Verification items for the finished model (mm, model axes). A direction names the side the tool comes from. Give positions to 0.01 mm unless a question says otherwise; leave off trailing zeros. Order: outer loops, then holes, each group sorted by start corner. A loop starts at its lowest first (then second) coordinate and runs counter-clockwise, first axis right, second up. Notation, with made-up numbers: M 83,-7 L 123,-7 A21 cw 123,-2 Z; hole C 36.25,11 d8. An arc over 180 degrees is marked long. Answer as a JSON object with one key per item and string values.
```python
from build123d import *

# Parameters (mm, degrees)
BOSS_EXTRUDE1_DEPTH = 50.8
FILLET1_R           = 2.54
FILLET2_R           = 2.54
SKETCH7_R           = 2.54
CUT_EXTRUDE1_DEPTH  = 50.8
SKETCH3_R           = 2.54
CUT_EXTRUDE2_DEPTH  = 50.8


with BuildPart() as part:
    # Sketch2 → Boss-Extrude1 (new body)
    with BuildSketch(Plane(origin=(0, 0, 0), x_dir=(1, 0, 0), z_dir=(0, 1, 0))):
        Polygon((-22.709183551, 14.294994846), (-22.709183551, -8.819005154), (-45.823183551, -8.819005154), (-45.823183551, -11.105005154), (-20.423183551, -11.105005154), (-20.423183551, 14.294994846), align=None)
    extrude(amount=BOSS_EXTRUDE1_DEPTH)

    # Fillet1
    fillet1_edges = [part.edges().sort_by_distance(p)[0] for p in [
        (-22.709183551, 25.4, 8.819005154),
    ]]
    fillet(fillet1_edges, radius=FILLET1_R)

    # Fillet2
    fillet2_edges = [part.edges().sort_by_distance(p)[0] for p in [
        (-20.423183551, 25.4, 11.105005154),
    ]]
    fillet(fillet2_edges, radius=FILLET2_R)

    # Sketch7 → Cut-Extrude1 (cut)
    with BuildSketch(Plane(origin=(0, 0, 8.819005154), x_dir=(-1, 0, 0), z_dir=(0, 0, -1))):
        with Locations((32.869183551, 38.1)):
            Circle(SKETCH7_R)
        with Locations((32.869183551, 12.7)):
            Circle(SKETCH7_R)
    extrude(amount=-CUT_EXTRUDE1_DEPTH, mode=Mode.SUBTRACT)

    # Sketch3 → Cut-Extrude2 (cut)
    with BuildSketch(Plane.ZY.offset(22.709183551)):
        with Locations((-1.340994846, 12.7)):
            Circle(SKETCH3_R)
        with Locations((-1.340994846, 38.1)):
            Circle(SKETCH3_R)
    extrude(amount=-CUT_EXTRUDE2_DEPTH, mode=Mode.SUBTRACT)


solid = part.part
```
Q1. Material ranges on L1, parallel to Y at x = -22.5, z = -1; L2, parallel to Z at x = -26.75, y = 32 (3 decimals); L3, parallel to X at y = 41, z = 4.75, recorded low to high.
Resolved:
{"L1": "y = 0 to 10.18, 15.22 to 35.58, 40.62 to 50.8", "L2": "z = 8.819 to 11.105", "L3": "x = -22.71 to -20.42"}
Q2. Tool access check on faces 1 (the face through (-21.58, 40.62, -1.67)), 2 (the face through (-22.709, 25, -4)). Record the directions out of +Z, -Z, +X, -X, +Y, -Y that give a thin tool (end or side, any length) a straight path to the whole face; none if there is none.
Resolved:
{"face 1": "+X, -X", "face 2": "-Z, -X, +Y, -Y"}
Q3. Section check A-A on y = 12.7. Record the cut outline in (x, z) (3 decimals), then the cut area to 3 significant figures.
Resolved:
{"outline": "M -45.823,8.819 L -35.409,8.819 L -35.409,11.105 L -45.823,11.105 Z; M -30.329,8.819 L -25.249,8.819 A2.54 cw -22.709,6.279 L -22.709,1.199 L -20.423,1.199 L -20.423,8.565 A2.54 ccw -22.963,11.105 L -30.329,11.105 Z; M -22.709,-14.295 L -20.423,-14.295 L -20.423,-3.881 L -22.709,-3.881 Z", "area": "87.7 mm²"}
Q4. Section check C-C on x = -43. Record the cut outline in (y, z) (3 decimals), then the cut area to 3 significant figures.
Resolved:
{"outline": "M 0,8.819 L 50.8,8.819 L 50.8,11.105 L 0,11.105 Z", "area": "116 mm²"}
Q5. Section check D-D on z = 2. Record the cut outline in (x, y).
Resolved:
{"outline": "M -22.71,0 L -20.42,0 L -20.42,50.8 L -22.71,50.8 Z"}
Q6. Release check for a two-part mould opening along Z. For faces 3 (the face through (-32.54, 15.22, 9.95)), 4 (the face through (-21.147, 25.756, 10.341)), 5 (the face through (-21.58, 15.22, -1.67)) record: +Z half, -Z half, draft (parallel to the pull), parting line (faces both ways), or undercut.
Resolved:
{"face 3": "draft", "face 4": "+Z half", "face 5": "undercut"}
Q7. Gauge pin test, flat ends, axial feed: pin 1 Ø8 at (x, z) = (-28.5, -10) entering from -Y; pin 2 Ø12 at (x, z) = (-24, -6) entering from -Y; pin 3 Ø12 at (x, y) = (-29, 23) entering from -Z; pin 4 Ø6 at (y, z) = (12.7, -1.34) entering from -X. Record the tip position at first contact, or that the pin passes through.
Resolved:
{"pin 1": "passes through", "pin 2": "stops at y = 0", "pin 3": "stops at z = 7.46", "pin 4": "stops at x = -22.71"}
Q8. Section check B-B on y = 23.5. Record the cut outline in (x, z) (3 decimals).
Resolved:
{"outline": "M -45.823,8.819 L -25.249,8.819 A2.54 cw -22.709,6.279 L -22.709,-14.295 L -20.423,-14.295 L -20.423,8.565 A2.54 ccw -22.963,11.105 L -45.823,11.105 Z"}
